Source: CAD feature listing. Evaluate the final solid. Frame: model axes, mm. A direction names the side the tool comes from. Give positions to 0.01 mm unless a question says otherwise; leave off trailing zeros. Order: outer loops, then holes, each group sorted by start corner. A loop starts at its lowest first (then second) coordinate and runs counter-clockwise, first axis right, second up.
1) Access query for faces 1 (the face through (-13, 5.7, 7)), 2 (the face through (9, 18, 7)), 3 (the face through (-20.715, 0.301, 7.098)). Directions: +Z, -Z, +X, -X, +Y, -Y. A direction counts if a zero-diameter tool reaches every point of the face in a straight line with its end or side. Return the directions, or none.
2) Material intervals for line 1 (Z direction, x = 16, y = 3.2); line 2 (Y direction, x = 0, z = 10.75); line 3 (X direction, y = 3, z = 8.5), sorted ascending.
3) Section A-A, the plane y = 20. Return loops of the section in (x, z), plus the area to 3 significant figures.
4) Section D-D, the plane z = 12.5. Return loops of the section in (x, y).
5) Draft query along X for faces 4 (the face through (21, 3, 7)), 5 (the face through (-0.521, 23.966, 6.902)), 6 (the face through (13, 5.7, 7)). Return one class per face: released by +X, released by -X, zero draft, split by the parting line, or undercut.
6) First-contact query: P1, Ø1, axis at x = -4, y = 21, coming from the -Z side; P2, Ø6.5, axis at x = 0, y = 20, coming from the +Z side; P3, Ø1.5, axis at x = 12, z = 4.5, coming from the +Y side; P4, Ø2, axis at y = 23, z = 12, coming from the -X side. Flat tips, straight axial feed; report the tip coordinate or a pass-through.
7) Section B-B, the plane z = 7. Return loops of the section in (x, y).
8) Section C-C, the plane x = 0. Return loops of the section in (y, z).
```python
from build123d import *

# Parameters (mm, degrees)
SKETCH_R     = 4
PAD_DEPTH    = 14
SKETCH001_R  = 2.75
POCKET_DEPTH = 5.7
FILLET_R     = 1.5
FILLET001_R  = 1


with BuildPart() as part:
    # Sketch → Pad (new body)
    with BuildSketch(Plane.XY):
        Polygon((-21, 0), (21, 0), (21, 5.7), (9, 5.7), (9, 33), (-9, 33), (-9, 5.7), (-21, 5.7), align=None)
        with Locations((0, 20)):
            Circle(SKETCH_R, mode=Mode.SUBTRACT)
    extrude(amount=PAD_DEPTH)

    # Sketch001 (on Face3 of Pad) → Pocket (cut)
    with BuildSketch(Plane(origin=(0, 5.7, 0), x_dir=(-1, 0, 0), z_dir=(0, 1, 0))):
        with Locations((-16, 7)):
            Circle(SKETCH001_R)
    pocket = extrude(amount=-POCKET_DEPTH, mode=Mode.SUBTRACT)

    # Mirrored: Pocket across Sketch001 V_Axis
    add(pocket.mirror(Plane(origin=(0, 5.7, 0), x_dir=(0, 1, 0), z_dir=(-1, 0, 0))), mode=Mode.SUBTRACT)

    # Fillet
    fillet_edges = [part.edges().sort_by_distance(p)[0] for p in [
        (21, 5.7, 7),
        (-21, 5.7, 7),
        (-9, 33, 7),
        (9, 33, 7),
    ]]
    fillet(fillet_edges, radius=FILLET_R)

    # Fillet001
    fillet001_edges = [part.edges().sort_by_distance(p)[0] for p in [
        (21, 0, 7),
        (-21, 0, 7),
    ]]
    fillet(fillet001_edges, radius=FILLET001_R)


solid = part.part
```
From the geometry:
1. face 1: +Z, -Z, -X, +Y
1. face 2: +Z, -Z, +X, +Y
1. face 3: +Z, -Z, -X, -Y
2. line 1: z = 0 to 4.25, 9.75 to 14
2. line 2: y = 0 to 16, 24 to 33
2. line 3: x = -21 to -18.3, -13.7 to 13.7, 18.3 to 21
3. outline: (-9, 0) - (-4, 0) - (-4, 14) - (-9, 14) - close; (4, 0) - (9, 0) - (9, 14) - (4, 14) - close
3. area: 140 mm2
4. outline: (-21, 1) arc R1 ccw to (-20, 0) - (20, 0) arc R1 ccw to (21, 1) - (21, 4.2) arc R1.5 ccw to (19.5, 5.7) - (9, 5.7) - (9, 31.5) arc R1.5 ccw to (7.5, 33) - (-7.5, 33) arc R1.5 ccw to (-9, 31.5) - (-9, 5.7) - (-19.5, 5.7) arc R1.5 ccw to (-21, 4.2) - close; hole circle Ø8 at (0, 20)
5. face 4: released by +X
5. face 5: undercut
5. face 6: zero draft
6. P1: stops at z = 0
6. P2: passes through
6. P3: stops at y = 5.7
6. P4: stops at x = -9
7. outline: (-21, 1) arc R1 ccw to (-20, 0) - (-18.75, 0) - (-18.75, 5.7) - (-19.5, 5.7) arc R1.5 ccw to (-21, 4.2) - close; (-13.25, 0) - (13.25, 0) - (13.25, 5.7) - (9, 5.7) - (9, 31.5) arc R1.5 ccw to (7.5, 33) - (-7.5, 33) arc R1.5 ccw to (-9, 31.5) - (-9, 5.7) - (-13.25, 5.7) - close; (18.75, 0) - (20, 0) arc R1 ccw to (21, 1) - (21, 4.2) arc R1.5 ccw to (19.5, 5.7) - (18.75, 5.7) - close; hole circle Ø8 at (0, 20)
8. outline: (0, 0) - (16, 0) - (16, 14) - (0, 14) - close; (24, 0) - (33, 0) - (33, 14) - (24, 14) - close
